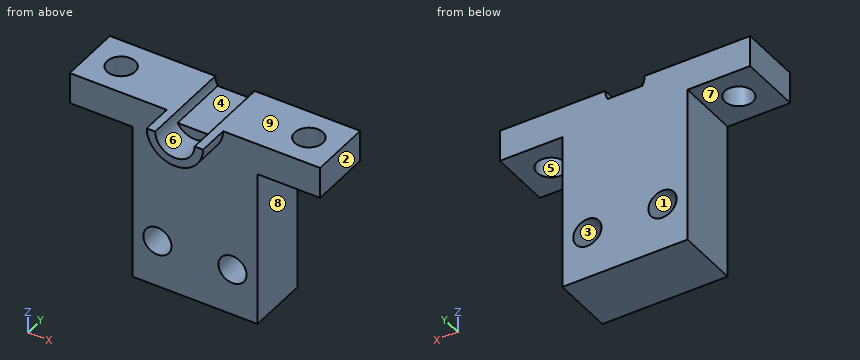
Autodesk Inventor part; units mm, degrees
ref_plane "YZ Plane" through (0, 0, 0) normal (1, 0, 0) x (0, 1, 0)
ref_plane "XZ Plane" through (0, 0, 0) normal (0, 1, 0) x (-1, 0, 0)
ref_plane "XY Plane" through (0, 0, 0) normal (0, 0, 1) x (1, 0, 0)
sketch "Sketch1" plane through (0, 0, 0) normal (0, 1, 0) x (-1, 0, 0)
  circle A0 centre (0, 0) radius 3.15
  line L0 (10, 0) -> (10, 30)
  line L1 (10, 30) -> (-10, 30)
  line L2 (-10, 30) -> (-10, 0)
  line L3 (10, -5) -> (10, -30)
  line L4 (10, -30) -> (-10, -30)
  line L5 (-10, -30) -> (-10, -5)
  line L6 (-10, 30) -> (-10, 15)
  line L7 (10, 30) -> (10, 15)
  line L8 (10, -30) -> (10, -15)
  line L9 (-10, -15) -> (-10, -30)
  line L10 (2.5151, -1.8965) -> (-2.5151, -1.8965)
  circle A1 centre (0, 0) radius 4.5
  line L11 (10, 0) -> (3.15, 0)
  line L12 (-3.15, 0) -> (-10, 0)
  line L13 (-10, 0) -> (-20, 0)
  line L14 (-20, 0) -> (-20, -5)
  line L15 (-20, -5) -> (-10, -5)
  line L16 (10, 0) -> (20, 0)
  line L17 (20, 0) -> (20, -5)
  line L18 (20, -5) -> (10, -5)
  line L19 (-4.5, 0) -> (-3.15, 0)
  line L20 (3.15, 0) -> (4.5, 0)
  circle A2 centre (6, 22.5) radius 2.25
  circle A3 centre (-5, 22.5) radius 2.25
  circle A4 centre (-6, -22.5) radius 2.25
  circle A5 centre (6, -22.5) radius 2.25
  line L21 (0, -1.8965) -> (0, -1.4965)
  line L22 (0, -1.4965) -> (-2.7718, -1.4965)
  line L23 (0, -1.4965) -> (2.7718, -1.4965)
  dimension "d0" = 6.3
  dimension "d6" = 15
  dimension "d34" = 9
  dimension "d35" = 10
  dimension "d36" = 5
  dimension "d37" = 10
  dimension "d38" = 5
  dimension "d43" = 4.5
  dimension "d44" = 4.5
  dimension "d45" = 4.5
  dimension "d46" = 4.5
  dimension "d59" = 0.4
extrude "Extrusion10" add sketch "Sketch1" along normal blind 10 contours L11 A1 L12 A0 | L11 L16 L17 L18 L3 L4 L5 L15 L14 L13 L12 A1 | A0 L10 picked at (3.9921, -0.5315)
extrude "Extrusion11" add sketch "Sketch1" against normal blind 5 contours L11 A1 L12 A0 picked at (3.9921, -0.5315)
sketch "Sketch3" plane through (3.15, 10, 0) normal (0, 0, 1) x (1, 0, 0)
  line L0 (16.85, 0) -> (16.85, -5)
  line L1 (16.85, -10) -> (16.85, 0)
  line L2 (16.85, -5) -> (11.85, -5)
  line L3 (-23.15, 0) -> (-23.15, -5)
  line L4 (-23.15, -10) -> (-23.15, 0)
  line L5 (-23.15, -5) -> (-18.15, -5)
  circle A0 centre (-18.15, -5) radius 2.25
  circle A1 centre (11.85, -5) radius 2.25
  point P0 (-3.15, -10)
  dimension "d51" = 5
  dimension "d52" = 5
  dimension "d53" = 5
  dimension "d54" = 5
  dimension "d55" = 4.5
  dimension "d56" = 4.5
extrude "Extrusion12" cut sketch "Sketch3" against normal blind 10
extrude "Extrusion13" add sketch "Sketch1" along normal blind 10 contours A0 L10 L21 L23 | L22 L21 L10 A0
properties part number "clip_to_shaft_holder"
Design review of the part built by this model. Coordinates are the model's own, in mm. Face numbers are marked on the shaded views. A direction names the side the tool comes from. Coordinates: 2 decimals unless noted, no trailing zeros. Loops run counter-clockwise (first coordinate to the right, second up) from the corner with the lowest first, then second, coordinate; pieces in that order, holes last. Notation, with made-up numbers: M 62,-36 L 105,-36 A20 ccw 105,-4 Z; hole C 77.25,48 d1. An arc over 180 degrees is marked long. Use one line per item in the form item = value.
(1) Consider section C-C (z = -22.5). Write out the cut boundary in (x, y), and give its area (3 significant figures).
Return value:
outline = M -10,0 L -8.25,0 L -8.25,10 L -10,10 Z; M -3.75,0 L 3.75,0 L 3.75,10 L -3.75,10 Z; M 8.25,0 L 10,0 L 10,10 L 8.25,10 Z
area = 110 mm2
(2) Clearance check with flat-ended pins moving along their axes: P1, Ø1.5, axis at x = -9, z = -7.5, coming from the -Y side; P2, Ø8, axis at x = 16.5, y = 6, coming from the -Z side; P3, Ø5, axis at y = 3, z = -15.5, coming from the +X side; P4, Ø2.5, axis at x = -6, z = -22.5, coming from the -Y side. State where each tip first meets the part, or that it passes through.
Return value:
P1 = 0
P2 = -5
P3 = 10
P4 = through
(3) For line 1 along Z through (x, y) = (-6, 3); line 2 along Y through (x, z) = (15, -3.1); line 3 along X through (y, z) = (6.25, -23.5), list the stretches that pass through material, from the lowest coordinate up. Write a range as from..to.
Return value:
line_1 = -30..-24.75, -20.25..0
line_2 = 0..2.75, 7.25..10
line_3 = -10..-8.02, -3.98..3.98, 8.02..10
(4) Consider section B-B (x = -15). Write out the cut boundary in (y, z).
Return value:
outline = M 0,-5 L 2.75,-5 L 2.75,0 L 0,0 Z; M 7.25,-5 L 10,-5 L 10,0 L 7.25,0 Z
(5) Consider section D-D (x = 0). Write out the cut boundary in (y, z).
Return value:
outline = M -5,-4.5 L 0,-4.5 L 0,-30 L 10,-30 L 10,-1.5 L 0,-1.5 L 0,-3.15 L -5,-3.15 Z
(6) For the marked faces 5, 6, 7, 8 and 9, list the 3-axis set-ups (+Z, -Z, +X, -X, +Y, -Y) from which the entire face can be reached by the end or side of a thin tool; tool diameter is ignored.
Return value:
face_5 = +Z, -Z
face_6 = +Z, -Y
face_7 = -Z, -X, +Y, -Y
face_8 = -Z, +X, +Y, -Y
face_9 = +Z, +X, -X, +Y, -Y
(7) Draft analysis for pull direction Z (two halves, no side actions). For the marked faces 1, 2, 3 and 4, state which applies: pulls with the +Z half, pulls with the -Z half, needs draft (parallel to the pull), parting line crosses it, or undercut.
Return value:
face_1 = undercut
face_2 = needs draft
face_3 = undercut
face_4 = pulls with the +Z half
(8) Consider section A-A (y = 5). Write out the cut boundary in (x, z), and give its area (3 significant figures).
Return value:
outline = M -20,-5 L -17.25,-5 L -17.25,0 L -20,0 Z; M -12.75,-5 L -10,-5 L -10,-30 L 10,-30 L 10,-5 L 12.75,-5 L 12.75,0 L 3.15,0 A3.15 cw 2.77,-1.5 L -2.77,-1.5 A3.15 cw -3.15,0 L -12.75,0 Z; M 17.25,-5 L 20,-5 L 20,0 L 17.25,0 Z; hole C -6,-22.5 d4.5; hole C 6,-22.5 d4.5
area = 614 mm2
